Source: CAD feature listing. Evaluate the final solid. Frame: model axes, mm. A direction names the side the tool comes from. Coordinates: 2 decimals unless noted, no trailing zeros. Order: outer loops, then holes, each group sorted by start corner. A loop starts at its lowest first (then second) coordinate and runs counter-clockwise, first axis right, second up. Notation, with made-up numbers: (74, 57) -> (132, 57) arc R13 cw to (132, 81) -> close; hole circle Ø9 at (15, 84). An arc over 180 degrees is marked (long way). Write each question's results on one line, items separated by ' | '. Start each with the question number.
Autodesk Inventor part; units mm, degrees
ref_plane "YZ Plane" through (0, 0, 0) normal (1, 0, 0) x (0, 1, 0)
ref_plane "XZ Plane" through (0, 0, 0) normal (0, 1, 0) x (-1, 0, 0)
ref_plane "XY Plane" through (0, 0, 0) normal (0, 0, 1) x (1, 0, 0)
sketch "Sketch1" plane through (0, 0, 0) normal (0, 0, 1) x (1, 0, 0)
  line L0 (0, 0) -> (600, 0)
  line L1 (100, -188) -> (500, -188)
  line L2 (500, -188) -> (500, -55)
  line L3 (500, -55) -> (600, -55)
  line L4 (600, -55) -> (600, 0)
  line L5 (100, -188) -> (100, -55)
  line L6 (0, -55) -> (0, 0)
  line L7 (0, -55) -> (100, -55)
  point P0 (300, -188)
  point P1 (300, 0)
  dimension "d0" = 600
  dimension "d1" = 188
  dimension "d2" = 400
  dimension "d3" = 133
extrude "Extrusion1" add sketch "Sketch1" along normal blind 10
sketch "Sketch2" plane through (0, 0, 10) normal (0, 0, 1) x (1, 0, 0)
  line L0 (600, 0) -> (0, 0)
  line L1 (500, -188) -> (100, -188)
  line L2 (600, 0) -> (300, 0)
  line L3 (300, 0) -> (300, -188)
  line L4 (300, -188) -> (600, -188)
  line L5 (600, -188) -> (600, 0)
extrude "Extrusion2" cut sketch "Sketch2" against normal through all
sketch "Sketch3" plane through (0, 0, 10) normal (0, 0, 1) x (1, 0, 0)
  circle A0 centre (10, -10) radius 2
  line L0 (300, 0) -> (0, 0)
  line L1 (0, 0) -> (0, -55)
  circle A1 centre (150, -10) radius 2
  circle A2 centre (290, -10) radius 2
  line L2 (300, -188) -> (300, 0)
  line L3 (10, -10) -> (290, -10) construction
  circle A3 centre (110, -178) radius 2
  line L4 (100, -55) -> (100, -188)
  line L5 (100, -188) -> (300, -188)
  circle A4 centre (290, -178) radius 2
  dimension "d8" = 4
  dimension "d9" = 10
  dimension "d10" = 10
  dimension "d11" = 4
  dimension "d12" = 4
  dimension "d13" = 10
  dimension "d14" = 4
  dimension "d15" = 10
  dimension "d16" = 10
  dimension "d17" = 4
  dimension "d18" = 10
  dimension "d19" = 10
extrude "Extrusion3" cut sketch "Sketch3" against normal through all
sketch "Sketch6" plane through (0, 0, 10) normal (0, 0, 1) x (1, 0, 0)
  line L0 (300, -31.5) -> (280, -31.5)
  line L1 (280, -31.5) -> (280, -156.5)
  line L2 (280, -156.5) -> (300, -156.5)
  line L3 (300, -156.5) -> (300, -31.5)
  line L4 (300, -188) -> (300, 0)
  point P0 (0, 0)
  point P1 (300, -94)
  dimension "d42" = 20
  dimension "d43" = 125
extrude "Extrusion6" cut sketch "Sketch6" against normal blind 5
sketch "Sketch7" plane through (0, 0, 5) normal (0, 0, 1) x (1, 0, 0)
  line L0 (290, -46.5) -> (290, -141.5) construction
  circle A0 centre (290, -46.5) radius 2.5
  circle A1 centre (290, -141.5) radius 2.5
  line L1 (300, -31.5) -> (300, -156.5)
  point P0 (0, 0)
  point P1 (290, -94)
  point P2 (300, -94)
  dimension "d46" = 5
  dimension "d47" = 5
  dimension "d48" = 10
  dimension "d49" = 95
extrude "Extrusion7" cut sketch "Sketch7" against normal through all
properties part number "SP001b" material "ABS Plastic"
(1) Line query: L1, parallel to X at y = -178, z = 5.25; L2, parallel to Y at x = 290, z = 3.95; L3, parallel to X at y = -10.5, z = 7. Output: solid intervals per line, ascending.
(2) Section A-A on z = 2. Return the cut outline in (x, y).
(3) Draft query along Y for faces 1 (the flat face through (290, -93, 5)), 2 (the flat face through (199, -188, 5)), 3 (the flat face through (100, -122, 5)), 4 (the flat face through (148, 0, 5)). Return one class per face: released by +Y, released by -Y, zero draft, split by the parting line, or undercut.
(4) First-contact query: P1, Ø6.5, axis at x = 290, y = -141.5, coming from the -Z side; P2, Ø1.5, axis at y = -79.5, z = 7.5, coming from the +X side; P3, Ø3, axis at x = 290, y = -178, coming from the +Z side; P4, Ø6.5, axis at x = 290, y = -46.5, coming from the +Z side. Flat tips, straight axial feed; report the tip coordinate or a pass-through.
(5) Section B-B on x = 66. Return the cut outline in (y, z).
(6) Reachability of faces 5 (the flat face through (49, -55, 5)), 6 (the flat face through (300, -93, 4)) from +Z, -Z, +X, -X, +Y, -Y: full face, straight path, thin tool, end or side. Return the list, or none.
(7) Section C-C on y = -69. Return the cut outline in (x, z), then the cut area to 3 significant figures.
Results list:
1) L1: x = 100 to 108, 112 to 288, 292 to 300 | L2: y = -188 to -180, -176 to -144, -139 to -49, -44 to -12, -8 to 0 | L3: x = 0 to 8.06, 11.94 to 148.06, 151.94 to 288.06, 291.94 to 300
2) outline: (0, -55) -> (100, -55) -> (100, -188) -> (300, -188) -> (300, 0) -> (0, 0) -> close; hole circle Ø4 at (10, -10); hole circle Ø4 at (110, -178); hole circle Ø4 at (150, -10); hole circle Ø5 at (290, -141.5); hole circle Ø5 at (290, -46.5); hole circle Ø4 at (290, -178); hole circle Ø4 at (290, -10)
3) face 1: undercut | face 2: released by -Y | face 3: zero draft | face 4: released by +Y
4) P1: stops at z = 0 | P2: stops at x = 280 | P3: passes through | P4: stops at z = 5
5) outline: (-55, 0) -> (0, 0) -> (0, 10) -> (-55, 10) -> close
6) face 5: +Z, -Z, -X, -Y | face 6: +Z, -Z, +X, +Y, -Y
7) outline: (100, 0) -> (300, 0) -> (300, 5) -> (280, 5) -> (280, 10) -> (100, 10) -> close | area: 1,900 mm²
